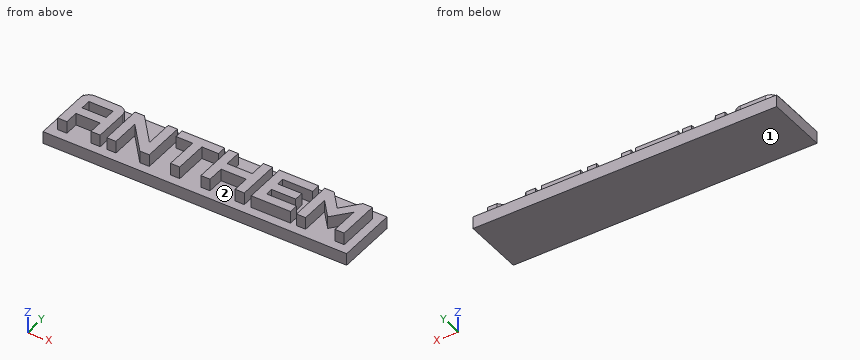
```python
from build123d import *

# Parameters (mm, degrees)
SKETCH1_W             = 1.983122363
SKETCH1_H             = 0.855133615
BOSS_EXTRUDE1_DEPTH   = 1
BOSS_EXTRUDE1_2_DEPTH = 1
BOSS_EXTRUDE1_3_DEPTH = 1
BOSS_EXTRUDE1_4_DEPTH = 1
BOSS_EXTRUDE1_5_DEPTH = 1
BOSS_EXTRUDE1_6_DEPTH = 1
SKETCH2_W             = 25
SKETCH2_H             = 5
BOSS_EXTRUDE2_DEPTH   = 1


with BuildPart() as part:
    # Sketch1 → Boss-Extrude1 (new body)
    with BuildSketch(Plane.XY):
        with BuildLine():
            Line((0.281997187, 0), (0.281997187, 2.780590717))
            add(Edge.make_bspline(
                [(0.281997187, 2.780590717), (0.283229244, 2.813026758), (0.285659888, 2.87701767), (0.304480904, 2.970500865), (0.334977853, 3.059415163), (0.377200617, 3.143135369), (0.43021619, 3.220013944), (0.490517367, 3.290502947), (0.560613021, 3.351341498), (0.637677118, 3.403898535), (0.721142214, 3.447362774), (0.810633683, 3.477327555), (0.904491397, 3.4964233), (0.968729628, 3.498794045), (1.00140647, 3.5)],
                knots=[0, 0, 0, 0, 1.032830424, 2.037602572, 3.024846489, 4.020164832, 5.014473951, 5.993861653, 6.967623515, 7.961932634, 8.960635615, 9.954944734, 10.959716882, 12, 12, 12, 12], degree=3))
            Line((1.00140647, 3.5), (3.05766526, 3.5))
            add(Edge.make_bspline(
                [(3.05766526, 3.5), (3.090103466, 3.498772386), (3.154098648, 3.496350507), (3.247550665, 3.477465492), (3.336681955, 3.447172624), (3.420051858, 3.403984292), (3.497130942, 3.350888644), (3.568573893, 3.290836996), (3.629457878, 3.219800158), (3.684008122, 3.143247784), (3.727453764, 3.059458406), (3.75985444, 2.970775725), (3.778237993, 2.876986116), (3.780732672, 2.813016144), (3.781997187, 2.780590717)],
                knots=[0, 0, 0, 0, 1.0309459, 2.033884719, 3.019327289, 4.016208014, 5.008702895, 5.991943608, 6.974449273, 7.975419069, 8.975722404, 9.966115281, 10.9690541, 12, 12, 12, 12], degree=3))
            Line((3.781997187, 2.780590717), (3.781997187, 0))
            Line((3.781997187, 0), (3.018284107, 0))
            Line((3.018284107, 0), (3.018284107, 1.127988748))
            Line((3.018284107, 1.127988748), (1.035161744, 1.127988748))
            Line((1.035161744, 1.127988748), (1.035161744, 0))
            Line((1.035161744, 0), (0.281997187, 0))
        make_face()
        with Locations((2.026722926, 2.313642757)):
            Rectangle(SKETCH1_W, SKETCH1_H, mode=Mode.SUBTRACT)
    extrude(amount=BOSS_EXTRUDE1_DEPTH)



with BuildPart() as body_2:
    # Sketch1 → Boss-Extrude1 2 (new body)
    with BuildSketch(Plane.XY):
        Polygon((4.32278481, 0), (4.32278481, 3.5), (5.100562588, 3.5), (7.059774965, 1.166666667), (7.059774965, 3.5), (7.82278481, 3.5), (7.82278481, 0), (7.045007032, 0), (5.075949367, 2.343178622), (5.075949367, 0), align=None)
    extrude(amount=BOSS_EXTRUDE1_2_DEPTH)


with BuildPart() as body_3:
    # Sketch1 → Boss-Extrude1 3 (new body)
    with BuildSketch(Plane.XY):
        Polygon((9.568917018, 0), (9.568917018, 2.741209564), (8.198312236, 2.741209564), (8.198312236, 3.5), (11.698312236, 3.5), (11.698312236, 2.741209564), (10.327707454, 2.741209564), (10.327707454, 0), align=None)
    extrude(amount=BOSS_EXTRUDE1_3_DEPTH)


with BuildPart() as body_4:
    # Sketch1 → Boss-Extrude1 4 (new body)
    with BuildSketch(Plane.XY):
        Polygon((12.068917018, 0), (12.068917018, 3.5), (12.822081575, 3.5), (12.822081575, 2.128691983), (14.888185654, 2.128691983), (14.888185654, 3.5), (15.641350211, 3.5), (15.641350211, 0), (14.888185654, 0), (14.888185654, 1.370604782), (12.822081575, 1.370604782), (12.822081575, 0), align=None)
    extrude(amount=BOSS_EXTRUDE1_4_DEPTH)


with BuildPart() as body_5:
    # Sketch1 → Boss-Extrude1 5 (new body)
    with BuildSketch(Plane.XY):
        Polygon((16.214486639, 0), (16.214486639, 3.5), (19.446554149, 3.5), (19.446554149, 2.741209564), (16.977496484, 2.741209564), (16.977496484, 2.128691983), (18.965541491, 2.128691983), (18.965541491, 1.370604782), (16.977496484, 1.370604782), (16.977496484, 0.758087201), (19.446554149, 0.758087201), (19.446554149, 0), align=None)
    extrude(amount=BOSS_EXTRUDE1_5_DEPTH)


with BuildPart() as body_6:
    # Sketch1 → Boss-Extrude1 6 (new body)
    with BuildSketch(Plane.XY):
        Polygon((19.940225035, 0), (19.940225035, 3.5), (20.718002813, 3.5), (21.904360056, 2.085091421), (23.085091421, 3.5), (23.867791842, 3.5), (23.867791842, 0), (23.109704641, 0), (23.109704641, 2.347398031), (21.904360056, 0.9092827), (20.693389592, 2.343178622), (20.693389592, 0), align=None)
    extrude(amount=BOSS_EXTRUDE1_6_DEPTH)


with BuildPart() as part_1:
    add(part.part)

    add(body_2.part)  # Boss-Extrude2 merges body 2

    add(body_3.part)  # Boss-Extrude2 merges body 3

    add(body_4.part)  # Boss-Extrude2 merges body 4

    add(body_5.part)  # Boss-Extrude2 merges body 5

    add(body_6.part)  # Boss-Extrude2 merges body 6
    # Sketch2 → Boss-Extrude2 (add)
    with BuildSketch(Plane(origin=(0, 0, 0), x_dir=(-1, 0, 0), z_dir=(0, 0, -1))):
        with Locations((-12.068917018, 1.75)):
            Rectangle(SKETCH2_W, SKETCH2_H)
    extrude(amount=BOSS_EXTRUDE2_DEPTH)


solid = part_1.part
```
Read the model definition and answer for the solid it produces. Units are mm, in the model's axes. Face numbers are marked on the shaded views. Give positions to 0.01 mm unless a question says otherwise; leave off trailing zeros. Order: outer loops, then holes, each group sorted by start corner. A loop starts at its lowest first (then second) coordinate and runs counter-clockwise, first axis right, second up. Notation, with made-up numbers: (27.25, 19.25) -> (42.25, 19.25) arc R11 cw to (42.25, 28.25) -> close; hole circle Ø8 at (49.25, -27). An arc over 180 degrees is marked (long way). One line per item, written item: value. Start each with the question number.
(1) Flat-ended cylindrical pins translate along their axes: P1, Ø0.8, axis at x = 23.5, z = 0.5, coming from the -Y side; P2, Ø0.5, axis at x = 18, z = 0.5, coming from the +Y side; P3, Ø0.5, axis at y = 0.5, z = 0.5, coming from the +X side. Find the tip coordinate at first contact, or state that the pin passes through.
(2) For a pull along X with two mould halves and no side action, classify the marked faces 1 and 2 as released by +X, released by -X, zero draft, split by the parting line, or undercut.
(3) The part is cut by section B-B (z = 0.55). State how many separate pieces and enclosed holes the cut face has, and give its area (3 significant figures).
(4) The part is cut by section D-D (x = 6). Determine the outline of the cut face in (y, z), and give its area (3 significant figures).
(5) Straight lines are drawn through the part: L1, parallel to Y at x = 18.25, z = 0.4; L2, parallel to Y at x = 10.25, z = 0.1; L3, parallel to Z at x = 8, y = 0.6. For each, find the intervals that lie inside material, in ascending order.
(6) The part is cut by section A-A (x = 8.75). Determine the outline of the cut face in (y, z), and give its area (3 significant figures).
(7) The part is cut by section C-C (y = 3.9). Determine the outline of the cut face in (x, z).
Taken from the geometry:
1. P1: y = 0
1. P2: y = 3.5
1. P3: x = 23.87
2. face 1: zero draft
2. face 2: undercut
3. separate pieces: 6
3. enclosed holes: 1
3. area: 43.4 mm^2
4. outline: (-0.75, -1) -> (4.25, -1) -> (4.25, 0) -> (2.43, 0) -> (2.43, 1) -> (1.24, 1) -> (1.24, 0) -> (-0.75, 0) -> close
4. area: 6.19 mm^2
5. L1: 0 to 0.76, 1.37 to 2.13, 2.74 to 3.5
5. L2: 0 to 3.5
5. L3: -1 to 0
6. outline: (-0.75, -1) -> (4.25, -1) -> (4.25, 0) -> (3.5, 0) -> (3.5, 1) -> (2.74, 1) -> (2.74, 0) -> (-0.75, 0) -> close
6. area: 5.76 mm^2
7. outline: (-0.43, -1) -> (24.57, -1) -> (24.57, 0) -> (-0.43, 0) -> close
